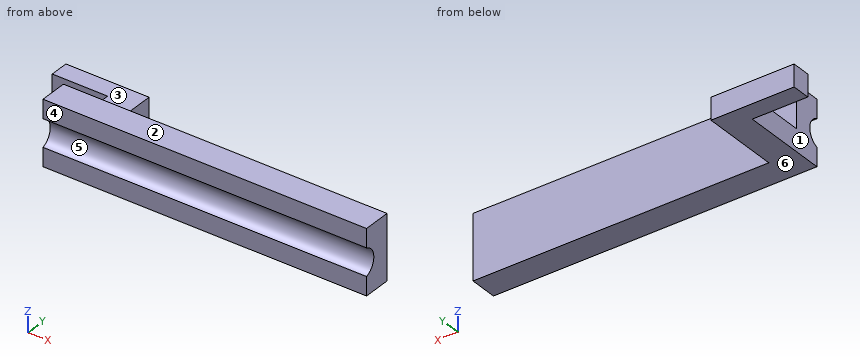
```python
from build123d import *

# Parameters (mm, degrees)
F0_W     = 88.9
F0_H     = 17.78
F1_DEPTH = 7.62
F2_R     = 3.9751
F3_DEPTH = 88.901
F4_W     = 7.62
F4_H     = 6.0452
F5_DEPTH = 21.59
F6_W     = 5.08
F6_H     = 6.0452
F7_DEPTH = 15.24


with BuildPart() as f1:
    # F0 (on Front) → F1 (new body)
    with BuildSketch(Plane.XZ):
        with Locations((-44.45, 8.89)):
            Rectangle(F0_W, F0_H)
    extrude(amount=F1_DEPTH)

    # F2 (on face) → F3 (cut, through all)
    with BuildSketch(Plane(origin=(-88.9, 0, 0), x_dir=(0, -1, 0), z_dir=(-1, 0, 0))):
        with Locations((8.89, 8.89)):
            Circle(F2_R)
    extrude(amount=-F3_DEPTH, mode=Mode.SUBTRACT)

    # F4 (on face) → F5 (join)
    with BuildSketch(Plane(origin=(0, 0, 0), x_dir=(-1, 0, 0), z_dir=(0, 1, 0))):
        with Locations((85.09, 3.0226)):
            Rectangle(F4_W, F4_H)
    extrude(amount=F5_DEPTH)

    # F6 (on face) → F7 (join)
    with BuildSketch(Plane(origin=(-88.9, 0, 0), x_dir=(0, -1, 0), z_dir=(-1, 0, 0))):
        with Locations((-19.05, 3.0226)):
            Rectangle(F6_W, F6_H)
    extrude(amount=F7_DEPTH)


solid = f1.part
```
Input: part model. Units: mm. Frame: model coordinates. Face numbers are marked on the shaded views. A direction names the side the tool comes from. Coordinates: 2 decimals unless noted, no trailing zeros. Order: outer loops, then holes, each group sorted by start corner. A loop starts at its lowest first (then second) coordinate and runs counter-clockwise, first axis right, second up. Notation, with made-up numbers: (21, 19.5) - (27, 19.5) arc R21 ccw to (27, 28.5) - close; hole circle Ø4 at (-10.5, 64.5). An arc over 180 degrees is marked (long way). Return JSON: item names as keys, results as strings.
Q1. First-contact query: pin 1 (3 mm diameter, centred on x = -59.5, z = 6, fed in from +Y); pin 2 (10 mm diameter, centred on x = -80, y = 14, fed in from +Z); pin 3 (9 mm diameter, centred on y = 4.5, z = 9, fed in from -X). Flat tips, straight axial feed; report the tip coordinate or a pass-through.
The answers:
{"pin 1": "stops at y = 0", "pin 2": "stops at z = 6.05", "pin 3": "stops at x = -88.9"}
Q2. Access query for the marked faces 1 and 2. Directions: +Z, -Z, +X, -X, +Y, -Y. A direction counts if a zero-diameter tool reaches every point of the face in a straight line with its end or side. Return the directions, or none.
The answers:
{"face 1": "+Z, -Z, -X, -Y", "face 2": "+Z, +X, -X, +Y, -Y"}
Q3. Draft query along Z for the marked faces 3, 4, 5 and 6. Return one class per face: +Z half, -Z half, draft (parallel to the pull), parting line (faces both ways), or undercut.
The answers:
{"face 3": "+Z half", "face 4": "draft", "face 5": "undercut", "face 6": "-Z half"}
Q4. Ray query, probe 1 along Y at (x, z) = (-52, 16); probe 2 along Z at (x, y) = (-16.5, -6); probe 3 along X at (y, z) = (-3.5, 9.25). Return the intervals inside material, ascending.
The answers:
{"probe 1": "y = -7.62 to 0", "probe 2": "z = 0 to 6.16, 11.62 to 17.78", "probe 3": "x = -88.9 to 0"}
Q5. Cut plane C-C (z = 7). Return loops of the section in (x, y).
The answers:
{"outline": "(-88.9, -5.39) - (0, -5.39) - (0, 0) - (-88.9, 0) - close"}
Q6. Cut plane A-A (x = -35). Return loops of the section in (y, z), then the cut area to 3 significant figures.
The answers:
{"outline": "(-7.62, 0) - (0, 0) - (0, 17.78) - (-7.62, 17.78) - (-7.62, 12.66) arc R3.98 cw to (-7.62, 5.12) - close", "area": "121 mm2"}
Q7. Cut plane B-B (y = 4.5). Return loops of the section in (x, z).
The answers:
{"outline": "(-88.9, 0) - (-81.28, 0) - (-81.28, 6.05) - (-88.9, 6.05) - close"}
